Read the model definition and answer for the solid it produces. Units are mm, in the model's axes. A direction names the side the tool comes from. Coordinates: 2 decimals unless noted, no trailing zeros. Order: outer loops, then holes, each group sorted by start corner. A loop starts at its lowest first (then second) coordinate and runs counter-clockwise, first axis right, second up. Notation, with made-up numbers: (24.5, -10) -> (74.5, -10) arc R12 cw to (74.5, -2) -> close; hole circle Ø3 at (10.25, -34). An arc over 180 degrees is marked (long way). Answer as a JSON object with one key per item and string values. Group by question number.
1) Given pin 1 (1.5 mm diameter, centred on x = 1.5, y = -1.5, fed in from -Z); pin 2 (2 mm diameter, centred on x = 1.5, z = -1, fed in from +Y); pin 3 (1.5 mm diameter, centred on x = 1, y = 1.5, fed in from +Z), each flat-ended and moving along its own axis, determine where each tip first touches the part or whether it passes through.
2) Section A-A on x = 2.9 is taken. Determine the outline of the cut face in (y, z).
3) Consider L1, parallel to Z at x = 1.35, y = -0.3; L2, parallel to X at y = -1.35, z = 1.45; L3, parallel to Z at x = 1.85, y = 0.7. Determine where each line is inside the solid, lowest interval first.
4) A tool of negligible diameter and unlimited length cuts with its end or side. For faces 1 (the flat face through (0, 1, -1)), 2 (the cylindrical face through (3.37, -0.45, 1.43)), from which of +Z, -Z, +X, -X, +Y, -Y can it reach the whole face along a straight path? Write none if from no direction.
from build123d import *

# Parameters (mm, degrees)
SKETCH3_W         = 0.79
SKETCH3_H         = 3.1
SKETCH4_W         = 0.395
SKETCH4_H         = 0.395
CIRPATTERN1_COUNT = 2
CIRPATTERN1_ANGLE = 90


with BuildPart() as part:
    # BodySke → Base-Revolve (revolve)
    with BuildSketch(Plane.XY, mode=Mode.PRIVATE) as base_revolve_sk:
        Polygon((0, 0), (0, 2.75), (0.45, 2.75), (1.7, 1.5), (5, 1.5), (5, 0), align=None)
    revolve(base_revolve_sk.sketch.rotate(Axis((-6.35, 0, 0), (1, 0, 0)), 90), axis=Axis((-6.35, 0, 0), (1, 0, 0)))  # turned: the seam where the file's is

    # Sketch3 → Cross section 0
    with BuildSketch(Plane.ZY):
        Rectangle(SKETCH3_W, SKETCH3_H)
    # Sketch4 → Cross section 1
    with BuildSketch(Plane.ZY.offset(-2.08)):
        Rectangle(SKETCH4_W, SKETCH4_H)
    cross = loft(mode=Mode.SUBTRACT)

    # CirPattern1: Cross ×2 about axis
    cirpattern1_axis = Axis((0, 0, 0), (1, 0, 0))
    for i in range(1, CIRPATTERN1_COUNT):
        add(cross.rotate(cirpattern1_axis, i * CIRPATTERN1_ANGLE / (CIRPATTERN1_COUNT - 1)), mode=Mode.SUBTRACT)


solid = part.part
Worked answers:
{
 "1": {"pin 1": "stops at z = -2.07", "pin 2": "stops at y = 2.56", "pin 3": "stops at z = 2.57"},
 "2": {"outline": "circle Ø3 at (0, 0)"},
 "3": {"L1": "z = -1.83 to -0.27, 0.27 to 1.83", "L2": "x = 0 to 1.22", "L3": "z = -1.33 to 1.33"},
 "4": {"face 1": "+Z, -Z, -X, +Y, -Y", "face 2": "+X"}
}
